For this review, use the dimensioned drawing (mm, ordinates from the lowest corner) and the shaded views. A direction names the side the tool comes from. Coordinates: 2 decimals unless noted, no trailing zeros. Loops run counter-clockwise (first coordinate to the right, second up) from the corner with the lowest first, then second, coordinate; pieces in that order, holes last. Notation, with made-up numbers: M 7,42 L 56,42 A12 ccw 56,62 Z; hole C 2,-33 d6. An arc over 180 degrees is marked long. Use CSV: the item, a comma, the result in double quotes. Start each with the question number.
1. Add section B-B, the plane z = 10. Write out the cut boundary in (x, y).
2. For L1, parallel to X at y = 9, z = 24; L2, parallel to Z at x = 30, y = 68; L3, parallel to Y at x = 52.5, z = 9.5, list the stretches that pass through material, from the lowest coordinate up.
3. Draft analysis for pull direction Y (two halves, no side actions). For the marked faces 3, 4 and 5, state which applies: +Y half, -Y half, draft (parallel to the pull), parting line (faces both ways), or undercut.
4. Add section C-C, the plane x = 50.5. Write out the cut boundary in (y, z).
5. Add section A-A, the plane x = 30. Write out the cut boundary in (y, z).
6. Clearance check with flat-ended pins moving along their axes: P1, Ø23, axis at x = 36, z = 37, coming from the -Y side; P2, Ø5.5, axis at x = 30, z = 10, coming from the -Y side. State where each tip first meets the part, or that it passes through.
7. Add section D-D, the plane y = 27.5. Write out the cut boundary in (x, z).
8. Tool access review of the marked faces 1 and 2: name each direction out of +Z, -Z, +X, -X, +Y, -Y from which nothing blocks a thin tool from reaching the whole face with its end or side.
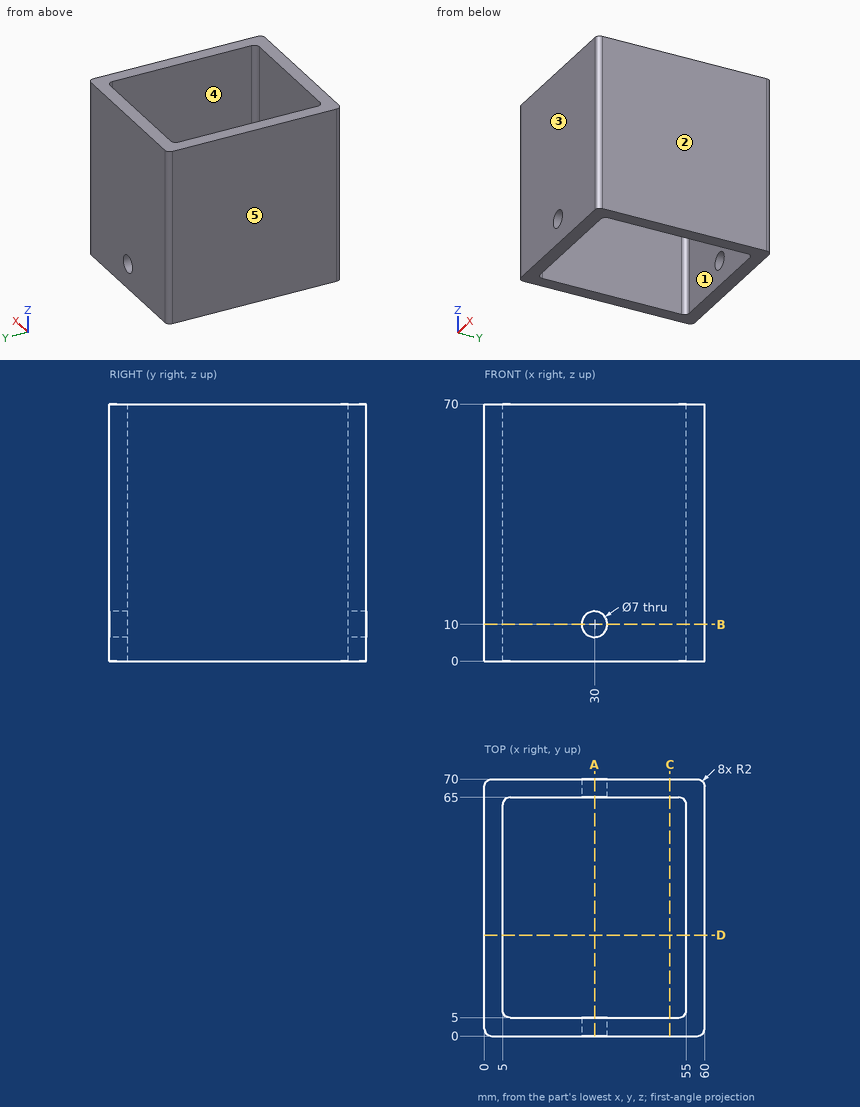
Computed:
1,outline,"M 0,2 A2 ccw 2,0 L 26.5,0 L 26.5,5 L 7,5 A2 cw 5,7 L 5,63 A2 cw 7,65 L 26.5,65 L 26.5,70 L 2,70 A2 ccw 0,68 Z; M 33.5,0 L 58,0 A2 ccw 60,2 L 60,68 A2 ccw 58,70 L 33.5,70 L 33.5,65 L 53,65 A2 cw 55,63 L 55,7 A2 cw 53,5 L 33.5,5 Z"
2,L1,"x = 0 to 5, 55 to 60"
2,L2,"z = 0 to 6.5, 13.5 to 70"
2,L3,"y = 0 to 5, 65 to 70"
3,face 3,"-Y half"
3,face 4,"undercut"
3,face 5,"draft"
4,outline,"M 0,0 L 5,0 L 5,70 L 0,70 Z; M 65,0 L 70,0 L 70,70 L 65,70 Z"
5,outline,"M 0,0 L 5,0 L 5,6.5 L 0,6.5 Z; M 0,13.5 L 5,13.5 L 5,70 L 0,70 Z; M 65,0 L 70,0 L 70,6.5 L 65,6.5 Z; M 65,13.5 L 70,13.5 L 70,70 L 65,70 Z"
6,P1,"stops at y = 0"
6,P2,"passes through"
7,outline,"M 0,0 L 5,0 L 5,70 L 0,70 Z; M 55,0 L 60,0 L 60,70 L 55,70 Z"
8,face 1,"+Z, -Z"
8,face 2,"+Z, -Z, +X, +Y, -Y"
